from build123d import *

# Parameters (mm, degrees)
F0_R     = 10.975
F1_DEPTH = 3.75
F2_R     = 7
F3_R     = 2.5


# Not quite as in the source:
# - a feature names something its author has since deleted; it is built from what else it names


with BuildPart() as f1:
    # F0 (on Top) → F1 (new body, symmetric)
    with BuildSketch(Plane.XY):
        Polygon((-5.4270925304, 33.057475201), (-10.8541850608, 23.657475201), (-25.9150670439, -2.4287376005), (-31.3421595743, -11.8287376005), (-25.9150670439, -21.2287376005), (-15.0608819831, -21.2287376005), (15.0608819831, -21.2287376005), (25.9150670439, -21.2287376005), (31.3421595743, -11.8287376005), (25.9150670439, -2.4287376005), (10.8541850608, 23.657475201), (5.4270925304, 33.057475201), align=None)
        Polygon((-16.9084028445, -5.6287376005), (-13.3288311755, -11.8287376005), (-16.9084028445, -18.0287376005), (-24.0675461825, -18.0287376005), (-27.6471178514, -11.8287376005), (-24.0675461825, -5.6287376005), align=None, mode=Mode.SUBTRACT)
        Circle(F0_R, mode=Mode.SUBTRACT)
        Polygon((24.0675461825, -5.6287376005), (27.6471178514, -11.8287376005), (24.0675461825, -18.0287376005), (16.9084028445, -18.0287376005), (13.3288311755, -11.8287376005), (16.9084028445, -5.6287376005), align=None, mode=Mode.SUBTRACT)
        Polygon((3.579571669, 29.857475201), (7.159143338, 23.657475201), (3.579571669, 17.457475201), (-3.579571669, 17.457475201), (-7.159143338, 23.657475201), (-3.579571669, 29.857475201), align=None, mode=Mode.SUBTRACT)
    extrude(amount=F1_DEPTH, both=True)

    # F2
    f2_edges = [f1.edges().sort_by_distance(p)[0] for p in [
        (31.34216, -11.828738, 0),
        (25.915067, -21.228738, 0),
        (-25.915067, -21.228738, 0),
        (-31.34216, -11.828738, 0),
        (-5.427093, 33.057475, 0),
        (5.427093, 33.057475, 0),
    ]]
    fillet(f2_edges, radius=F2_R)

    # F3
    f3_edges = [f1.edges().sort_by_distance(p)[0] for p in [
        (-18.384626, 10.614369, -3.75),
        (-7.447818, 29.557475, 0),
        (-29.321434, -8.328738, 0),
        (-18.384626, 10.614369, 3.75),
    ]]
    fillet(f3_edges, radius=F3_R)


solid = f1.part
The model under review builds one solid part; all positions refer to its coordinate system, in mm. A direction names the side the tool comes from. Coordinates: 2 decimals unless noted, no trailing zeros. Write each loop counter-clockwise with the first axis right and the second up, starting at its lowest first coordinate (ties: lowest second). Pieces come first, ordered by that corner, then holes. Notation, with made-up numbers: (58, 73) -> (101, 73) arc R33 ccw to (101, 108) -> close; hole circle Ø10 at (58.25, 4.5). An arc over 180 degrees is marked (long way). Answer in a Markdown table with one row per item.
1. Clearance check with flat-ended pins moving along their axes: pin 1 Ø2 at (x, z) = (1.5, 2) entering from +Y; pin 2 Ø2 at (y, z) = (25.5, 0) entering from -X; pin 3 Ø2 at (x, z) = (20, 0) entering from +Y; pin 4 Ø3 at (x, z) = (9, 1) entering from +Y. State where each tip first meets the part, or that it passes through.
Answers below:
| item | result |
|---|---|
| pin 1 | stops at y = 33.06 |
| pin 2 | stops at x = -10.37 |
| pin 3 | stops at y = 9.55 |
| pin 4 | stops at y = 29.47 |
2. We need section B-B, the plane z = -0.25. Give the number of separate pieces and of enclosed holes in the cut face, and give its area (3 significant figures).
Answers below:
| item | result |
|---|---|
| separate pieces | 1 |
| enclosed holes | 4 |
| area | 1,390 mm^2 |
3. For faces 1 (the cylindrical face through (28.021, -16.155, -2.998)), 2 (the flat face through (0, 29.857, 0)), list the 3-axis set-ups (+Z, -Z, +X, -X, +Y, -Y) from which the entire face can be reached by the end or side of a thin tool; tool diameter is ignored.
Answers below:
| item | result |
|---|---|
| face 1 | -Z, +X, -Y |
| face 2 | +Z, -Z |
4. Draft analysis for pull direction X (two halves, no side actions). For faces 3 (the cylindrical face through (-0.019, 32.345, 2.998)), 4 (the cylindrical face through (-28, -16.19, -3)), 5 (the flat face through (25.88, -14.89, 0.05)), state which applies: +X half, -X half, draft (parallel to the pull), parting line (faces both ways), or undercut.
Answers below:
| item | result |
|---|---|
| face 3 | draft |
| face 4 | -X half |
| face 5 | undercut |
5. We need section A-A, the plane x = 0. State the section outline as (y, z) points (3 decimals).
Answers below:
| item | result |
|---|---|
| outline | (-21.229, -1.25) arc R2.5 ccw to (-18.729, -3.75) -> (-10.975, -3.75) -> (-10.975, 3.75) -> (-18.729, 3.75) arc R2.5 ccw to (-21.229, 1.25) -> close; (10.975, -3.75) -> (17.457, -3.75) -> (17.457, 3.75) -> (10.975, 3.75) -> close; (29.857, -3.75) -> (30.557, -3.75) arc R2.5 ccw to (33.057, -1.25) -> (33.057, 1.25) arc R2.5 ccw to (30.557, 3.75) -> (29.857, 3.75) -> close |
6. Wall thickness on probe 1 along Y at (x, z) = (0, 0.25) (3 decimals); probe 2 along X at (y, z) = (-9, -3.25); probe 3 along Y at (x, z) = (5.5, 0.75): over which ranges is each line inside the solid? List them lowest first. Write a range as [from, to].
Answers below:
| item | result |
|---|---|
| probe 1 | y = [-21.229, -10.975], [10.975, 17.457], [29.857, 33.057] |
| probe 2 | x = [-28.55, -26.01], [-14.96, -6.28], [6.28, 14.96], [26.01, 28.55] |
| probe 3 | y = [-21.23, -9.5], [9.5, 20.78], [26.53, 31.72] |
